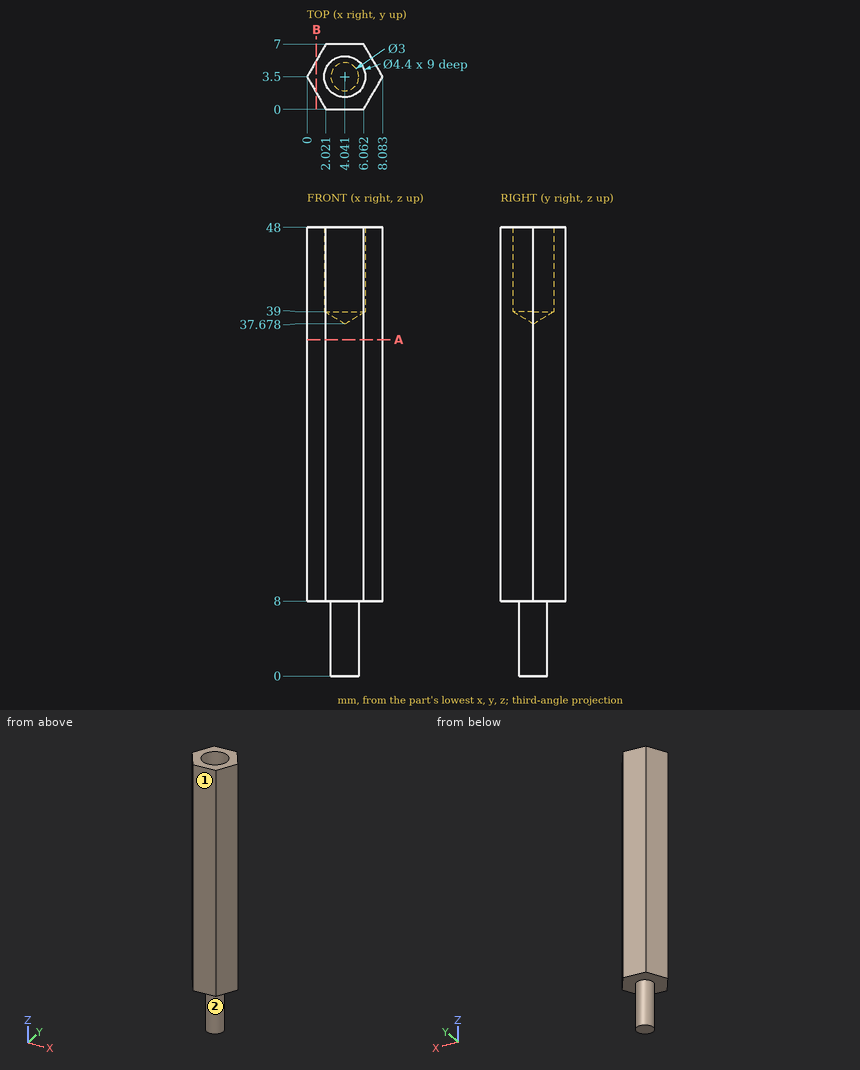
The figure shows three views and two pictorial views of one solid part (mm, origin at its lowest corner). Answer the questions. A direction names the side the tool comes from. Give positions to 0.01 mm unless a question says otherwise; leave off trailing zeros. Order: outer loops, then holes, each group sorted by start corner. A loop starts at its lowest first (then second) coordinate and runs counter-clockwise, first axis right, second up. Notation, with made-up numbers: (-24, 3.25) - (-8, 3.25) arc R28 ccw to (-8, 26.25) - close; hole circle Ø5 at (64, -5). An arc over 180 degrees is marked (long way). Answer as CSV lines item,"result".
Q1. A cutting plane is placed at B-B, the plane x = 1. Determine the outline of the cut face in (y, z).
Answer key:
outline,"(1.77, 8) - (5.23, 8) - (5.23, 48) - (1.77, 48) - close"
Q2. Straight lines are drawn through the part: L1, parallel to X at y = 3.5, z = 42.5; L2, parallel to Y at x = 4.25, z = 46; L3, parallel to Z at x = 3.5, y = 6. For each, find the intervals that lie inside material, in ascending order.
Answer key:
L1,"x = 0 to 1.84, 6.24 to 8.08"
L2,"y = 0 to 1.31, 5.69 to 7"
L3,"z = 8 to 48"
Q3. A cutting plane is placed at A-A, the plane z = 36. Determine the outline of the cut face in (x, y).
Answer key:
outline,"(0, 3.5) - (2.02, 0) - (6.06, 0) - (8.08, 3.5) - (6.06, 7) - (2.02, 7) - close"
Q4. Which of the six approach directions +Z, -Z, +X, -X, +Y, -Y give full straight-line access (tool end or side, diameter ignored) to the marked faces 1 and 2?
Answer key:
face 1,"+Z, -Z, +X, -X, -Y"
face 2,"-Z"
